```python
from build123d import *

# Parameters (mm, degrees)
F0_R     = 13.586014
F0_R_2   = 1.75
F1_DEPTH = 1.5
F2_DEPTH = 13
F3_DEPTH = 19


with BuildPart() as f1:
    # F0 (on Top) → F1 (new body)
    with BuildSketch(Plane.XY):
        with BuildLine():
            Line((43.291877, 24.555553), (22.56174, 24.555553))
            Line((22.56174, 24.555553), (22.56174, -5.444447))
            Line((22.56174, -5.444447), (24.640569, -6.751582))
            Line((24.640569, -6.751582), (31.699486, -11.190116))
            Line((31.699486, -11.190116), (33.062977, -12.047457))
            ThreePointArc((33.062977, -12.047457), (37.919879, -14.173764), (43.186607, -14.783891))
            ThreePointArc((43.186607, -14.783891), (48.465497, -14.09159), (53.365348, -12.008945))
            ThreePointArc((53.365348, -12.008945), (57.132258, -9.090982), (60.086993, -5.352845))
            ThreePointArc((60.086993, -5.352845), (62.961704, 4.923251), (60.047767, 15.188294))
            ThreePointArc((60.047767, 15.188294), (57.289995, 18.70438), (53.809777, 21.507281))
            ThreePointArc((53.809777, 21.507281), (48.767235, 23.778121), (43.291877, 24.555553))
        make_face()
        with Locations((43.186607, 3.091027)):
            Circle(F0_R, mode=Mode.SUBTRACT)
        with Locations((43.186607, 3.091027)):
            Circle(F0_R)
        with BuildLine():
            Line((31.699486, -11.190116), (24.640569, -6.751582))
            Line((24.640569, -6.751582), (22.912271, -11.682871))
            ThreePointArc((22.912271, -11.682871), (23.949593, -14.903245), (27.330435, -14.773852))
            Line((27.330435, -14.773852), (31.699486, -11.190116))
        make_face()
        with Locations((25.554683, -12.608973)):
            Circle(F0_R_2, mode=Mode.SUBTRACT)
        with BuildLine():
            Line((62.771435, -11.486311), (60.086993, -5.352845))
            ThreePointArc((60.086993, -5.352845), (57.132258, -9.090982), (53.365348, -12.008945))
            Line((53.365348, -12.008945), (58.845684, -15.056129))
            ThreePointArc((58.845684, -15.056129), (62.090115, -14.680554), (62.771435, -11.486311))
        make_face()
        with Locations((60.206356, -12.608973)):
            Circle(F0_R_2, mode=Mode.SUBTRACT)
        with BuildLine():
            Line((58.947953, 24.092311), (53.809777, 21.507281))
            ThreePointArc((53.809777, 21.507281), (57.289995, 18.70438), (60.047767, 15.188294))
            Line((60.047767, 15.188294), (62.693522, 20.304946))
            ThreePointArc((62.693522, 20.304946), (62.197209, 23.559911), (58.947953, 24.092311))
        make_face()
        with Locations((60.206356, 21.591027)):
            Circle(F0_R_2, mode=Mode.SUBTRACT)
    extrude(amount=F1_DEPTH)

    # F0 (on Top) → F2 (join)
    with BuildSketch(Plane.XY):
        with BuildLine():
            Line((31.699486, -11.190116), (24.640569, -6.751582))
            Line((24.640569, -6.751582), (22.912271, -11.682871))
            ThreePointArc((22.912271, -11.682871), (23.949593, -14.903245), (27.330435, -14.773852))
            Line((27.330435, -14.773852), (31.699486, -11.190116))
        make_face()
        with Locations((25.554683, -12.608973)):
            Circle(F0_R_2, mode=Mode.SUBTRACT)
        with BuildLine():
            Line((62.771435, -11.486311), (60.086993, -5.352845))
            ThreePointArc((60.086993, -5.352845), (57.132258, -9.090982), (53.365348, -12.008945))
            Line((53.365348, -12.008945), (58.845684, -15.056129))
            ThreePointArc((58.845684, -15.056129), (62.090115, -14.680554), (62.771435, -11.486311))
        make_face()
        with Locations((60.206356, -12.608973)):
            Circle(F0_R_2, mode=Mode.SUBTRACT)
        with BuildLine():
            Line((58.947953, 24.092311), (53.809777, 21.507281))
            ThreePointArc((53.809777, 21.507281), (57.289995, 18.70438), (60.047767, 15.188294))
            Line((60.047767, 15.188294), (62.693522, 20.304946))
            ThreePointArc((62.693522, 20.304946), (62.197209, 23.559911), (58.947953, 24.092311))
        make_face()
        with Locations((60.206356, 21.591027)):
            Circle(F0_R_2, mode=Mode.SUBTRACT)
    extrude(amount=F2_DEPTH)

    # F0 (on Top) → F3 (join)
    with BuildSketch(Plane.XY):
        with BuildLine():
            Line((43.291877, 24.555553), (22.56174, 24.555553))
            Line((22.56174, 24.555553), (22.56174, -5.444447))
            Line((22.56174, -5.444447), (24.640569, -6.751582))
            Line((24.640569, -6.751582), (31.699486, -11.190116))
            Line((31.699486, -11.190116), (33.062977, -12.047457))
            ThreePointArc((33.062977, -12.047457), (37.919879, -14.173764), (43.186607, -14.783891))
            ThreePointArc((43.186607, -14.783891), (48.465497, -14.09159), (53.365348, -12.008945))
            ThreePointArc((53.365348, -12.008945), (57.132258, -9.090982), (60.086993, -5.352845))
            ThreePointArc((60.086993, -5.352845), (62.961704, 4.923251), (60.047767, 15.188294))
            ThreePointArc((60.047767, 15.188294), (57.289995, 18.70438), (53.809777, 21.507281))
            ThreePointArc((53.809777, 21.507281), (48.767235, 23.778121), (43.291877, 24.555553))
        make_face()
        with Locations((43.186607, 3.091027)):
            Circle(F0_R, mode=Mode.SUBTRACT)
    extrude(amount=F3_DEPTH)


solid = f1.part
```
Could you check a few things on this model? Use its own coordinates, in mm. A direction names the side the tool comes from. Round coordinates to 2 decimals unless told otherwise and drop trailing zeros. Order: outer loops, then holes, each group sorted by start corner. A loop starts at its lowest first (then second) coordinate and runs counter-clockwise, first axis right, second up. Notation, with made-up numbers: M -21,84.5 L 27,84.5 A10 cw 27,88.5 Z; hole C 54,-11.75 d4. An arc over 180 degrees is marked long. One line per question, with ' | ' between items. Start each with the question number.
(1) Thinking about a two-plate mould opening in X: for faces 5 (the face through (23.79, -9.18, 6.41)), 6 (the face through (61.448, -8.463, 6.409)), 7 (the face through (27, -11, 13)), 8 (the face through (56.067, -13.511, 6.409)), which applies, +X half, -X half, draft (parallel to the pull), parting line (faces both ways), or undercut?
(2) For faces 1 (the face through (56.415, 22.818, 6.409)), 2 (the face through (29.48, -13.01, 6.41)), 3 (the face through (43, 3, 1.5)), 4 (the face through (59, -10, 13)), which set-ups out of +Z, -Z, +X, -X, +Y, -Y let a thin tool reach every point of the face, with its end or its side?
(3) For P1, Ø3, axis at y = 17, z = 6.5, coming from the +X side; P2, Ø8, axis at x = 52.5, z = 6, coming from the +Y side; P3, Ø9.5, axis at x = 25, y = -13, coming from the +Z side, each with a flat end and sliding along its axis, tell me the tip position at first contact or that it passes through.
(4) Suppose I cut it at D-D on z = 2. List the corners of the cut face in (x, y) for me, then the cut area to 3 significant figures.
(5) Suppose I cut it at C-C on y = 8. List the corners of the cut face in (x, z) for me.
(6) Suppose I cut it at A-A on x = 42.5. List the corners of the cut face in (y, z) for me, then the cut area to 3 significant figures.
(7) Please list where these lines run through material, in increasing order: line 1 along Z through (x, y) = (31, -11); line 2 along X through (y, z) = (-11.5, 11); line 3 along X through (y, z) = (9.5, 16).
(8) Suppose I cut it at B-B on z = 17.5. List the corners of the cut face in (x, y) for me.
Geometry results:
1) face 5: -X half | face 6: +X half | face 7: draft | face 8: undercut
2) face 1: +Z, -Z, +Y | face 2: +Z, -Z, -Y | face 3: +Z | face 4: +Z, +X, -Y
3) P1: x = 61.76 | P2: y = 23.85 | P3: z = 13
4) outline: M 22.56,-5.44 L 24.64,-6.75 L 22.91,-11.68 A2.8 ccw 27.33,-14.77 L 31.7,-11.19 L 33.06,-12.05 A17.9 ccw 43.19,-14.78 A19.67 ccw 53.37,-12.01 L 58.85,-15.06 A2.8 ccw 62.77,-11.49 L 60.09,-5.35 A19.67 ccw 60.05,15.19 L 62.69,20.3 A2.8 ccw 58.95,24.09 L 53.81,21.51 A19.67 ccw 43.29,24.56 L 22.56,24.56 Z; hole C 25.55,-12.61 d3.5; hole C 43.19,3.09 d27.17; hole C 60.21,-12.61 d3.5; hole C 60.21,21.59 d3.5 | area: 879 mm²
5) outline: M 22.56,0 L 62.71,0 L 62.71,19 L 55.85,19 L 55.85,1.5 L 30.52,1.5 L 30.52,19 L 22.56,19 Z
6) outline: M -14.79,0 L 24.56,0 L 24.56,19 L 16.66,19 L 16.66,1.5 L -10.48,1.5 L -10.48,19 L -14.79,19 Z | area: 273 mm²
7) line 1: 0 to 13 | line 2: 22.98 to 24.2, 26.91 to 31.32, 32.19 to 58.85, 61.56 to 62.78 | line 3: 22.56 to 31.21, 55.17 to 62.41
8) outline: M 22.56,-5.44 L 24.64,-6.75 L 31.7,-11.19 L 33.06,-12.05 A17.9 ccw 43.19,-14.78 A19.67 ccw 53.37,-12.01 A19.67 ccw 60.09,-5.35 A19.67 ccw 60.05,15.19 A19.67 ccw 53.81,21.51 A19.67 ccw 43.29,24.56 L 22.56,24.56 Z; hole C 43.19,3.09 d27.17
